from build123d import *

# Parameters (mm, degrees)
F1_DEPTH = 5.588
F2_DEPTH = 4.826


with BuildPart() as f1:
    # F0 (on Right) → F1 (new body)
    with BuildSketch(Plane.YZ):
        with BuildLine():
            Line((-20.567739, 0.302803), (-20.567739, 5.372244))
            ThreePointArc((-20.567739, 5.372244), (-24.780512, 3.122693), (-25.254471, -1.629496))
            Line((-25.254471, -1.629496), (-24.99502, -1.522527))
            Line((-24.99502, -1.522527), (-20.567739, 0.302803))
        make_face()
        Polygon((20.567561, 5.372244), (-0.006439, 5.372244), (-20.567739, 5.372244), (-20.567739, 0.302803), (20.567561, 0.302803), align=None)
        with BuildLine():
            ThreePointArc((25.255113, -1.627505), (24.779735, 3.123587), (20.567561, 5.372244))
            Line((20.567561, 5.372244), (20.567561, 0.302803))
            Line((20.567561, 0.302803), (25.000183, -1.522527))
            Line((25.000183, -1.522527), (25.255113, -1.627505))
        make_face()
    extrude(amount=-F1_DEPTH)

    # F0 (on Right) → F2 (join)
    with BuildSketch(Plane.YZ):
        Polygon((20.567561, 0.302803), (-20.567739, 0.302803), (-24.99502, -1.522527), (-15.208358, -9.628492), (15.210344, -9.628492), (25.000183, -1.522527), align=None)
    extrude(amount=-F2_DEPTH)


solid = f1.part
Read the model definition and answer for the solid it produces. Units are mm, in the model's axes. Coordinates: 2 decimals unless noted, no trailing zeros. Order: outer loops, then holes, each group sorted by start corner. A loop starts at its lowest first (then second) coordinate and runs counter-clockwise, first axis right, second up. Notation, with made-up numbers: (35.5, 57.25) - (41.5, 57.25) arc R23 cw to (41.5, 94.25) - close; hole circle Ø4 at (72.25, 16.5). An arc over 180 degrees is marked (long way). Use one line per item in the form item = value.
(1) Straight lines are drawn through the part: L1, parallel to X at y = 7, z = -8; L2, parallel to Z at x = -5.2, y = -11; L3, parallel to Z at x = -1.4, y = 22.5. For each, find the intervals that lie inside material, in ascending order.
Computed values:
L1 = -4.83 to 0
L2 = 0.3 to 5.37
L3 = -3.59 to 4.99
(2) Given pin 1 Ø8 at (y, z) = (5.5, -4.5) entering from -X, flat-ended and moving along its own axis, determine where the tip first touches the part or whether it passes through.
Computed values:
pin_1 = -4.83
(3) Section C-C, the plane z = -0.5 is taken. Give the vertices of the cut face in (x, y).
Computed values:
outline = (-5.59, -25.57) - (0, -25.57) - (0, 25.57) - (-5.59, 25.57) - (-5.59, 22.52) - (-4.83, 22.52) - (-4.83, -22.51) - (-5.59, -22.51) - close
(4) Section A-A, the plane x = -2.55 is taken. Give the vertices of the cut face in (y, z).
Computed values:
outline = (-25.25, -1.63) - (-25, -1.52) - (-15.21, -9.63) - (15.21, -9.63) - (25, -1.52) - (25.26, -1.63) arc R5.07 ccw to (20.57, 5.37) - (-20.57, 5.37) arc R5.07 ccw to start
(5) For a pull along Y with two mould halves and no side action, classify faces 1 (the face through (-2.75, -24.74, 3.18)), 2 (the face through (-4.826, 0, -5)), 3 (the face through (-2.755, 24.818, 3.065)), 4 (the face through (-3, 0, 5.372)) as pulls with the +Y half, pulls with the -Y half, needs draft (parallel to the pull), parting line crosses it, or undercut.
Computed values:
face_1 = pulls with the -Y half
face_2 = undercut
face_3 = pulls with the +Y half
face_4 = needs draft
(6) Section B-B, the plane y = -1 is taken. Give the vertices of the cut face in (x, z), then the cut area to 3 significant figures.
Computed values:
outline = (-5.59, 0.3) - (-4.83, 0.3) - (-4.83, -9.63) - (0, -9.63) - (0, 5.37) - (-5.59, 5.37) - close
area = 76.3 mm²
(7) Section D-D, the plane y = -22 is taken. Give the vertices of the cut face in (x, z).
Computed values:
outline = (-5.59, -0.29) - (-4.83, -0.29) - (-4.83, -4) - (0, -4) - (0, 5.17) - (-5.59, 5.17) - close
